Input: part model. Units: mm. Frame: model coordinates. A direction names the side the tool comes from. Round coordinates to 2 decimals unless told otherwise and drop trailing zeros. Order: outer loops, then holes, each group sorted by start corner. A loop starts at its lowest first (then second) coordinate and runs counter-clockwise, first axis right, second up. Notation, with made-up numbers: (30.25, 5.25) -> (50.25, 5.25) arc R19 ccw to (50.25, 27.25) -> close; hole circle Ø5 at (-24, 6). An arc over 180 degrees is marked (long way). Use a Markdown table: item, result.
from build123d import *

# Parameters (mm, degrees)
F0_W     = 2082.8
F0_H     = 914.4
F1_DEPTH = 25.4
F2_W     = 38.1
F2_H     = 88.9
F3_DEPTH = 2082.8
F4_W     = 38.1
F4_H     = 88.9
F5_DEPTH = 838.2
F6_W     = 88.9
F6_H     = 38.1
F7_DEPTH = 1143


# Not quite as in the source:
# - a feature names something its author has since deleted; it is built from what else it names


with BuildPart() as f1:
    # F0 (on Top) → F1 (new body)
    with BuildSketch(Plane.XY):
        with Locations((1041.4, -457.2)):
            Rectangle(F0_W, F0_H)
    extrude(amount=F1_DEPTH)

    # F2 (on face) → F3 (join, through all)
    with BuildSketch(Plane.YZ.offset(2082.8)):
        with Locations((-895.35, -44.45)):
            Rectangle(F2_W, F2_H)
        with Locations((-19.05, -44.45)):
            Rectangle(F2_W, F2_H)
    extrude(amount=-F3_DEPTH)

    # F4 (on face) → F5 (join, through all)
    with BuildSketch(Plane.XZ.offset(38.1)):
        with Locations((19.05, -44.45)):
            Rectangle(F4_W, F4_H)
        with Locations((2063.75, -44.45)):
            Rectangle(F4_W, F4_H)
    extrude(amount=F5_DEPTH)

    # F6 (on face) → F7 (join)
    with BuildSketch(Plane(origin=(0, 0, 0), x_dir=(1, 0, 0), z_dir=(0, 0, -1))):
        with Locations((82.55, 857.25)):
            Rectangle(F6_W, F6_H)
        with Locations((82.55, 57.15)):
            Rectangle(F6_W, F6_H)
        with Locations((2000.25, 57.15)):
            Rectangle(F6_W, F6_H)
        with Locations((2000.25, 857.25)):
            Rectangle(F6_W, F6_H)
    extrude(amount=F7_DEPTH)


solid = f1.part
1) Pull-direction query (Y, two-part tool) for faces 1 (the flat face through (2000, -38.1, -609)), 2 (the flat face through (2082.8, -464, -31)), 3 (the flat face through (82, -76.2, -563)), 4 (the flat face through (2044.7, -452, -45)); classes: +Y half, -Y half, draft (parallel to the pull), parting line (faces both ways), or undercut.
Results found:
| item | result |
|---|---|
| face 1 | +Y half |
| face 2 | draft |
| face 3 | undercut |
| face 4 | undercut |
2) Cut plane A-A on z = -650. Return loops of the section in (x, y), and give its area (3 significant figures).
Results found:
| item | result |
|---|---|
| outline | (38.1, -876.3) -> (127, -876.3) -> (127, -838.2) -> (38.1, -838.2) -> close; (38.1, -76.2) -> (127, -76.2) -> (127, -38.1) -> (38.1, -38.1) -> close; (1955.8, -876.3) -> (2044.7, -876.3) -> (2044.7, -838.2) -> (1955.8, -838.2) -> close; (1955.8, -76.2) -> (2044.7, -76.2) -> (2044.7, -38.1) -> (1955.8, -38.1) -> close |
| area | 13,500 mm² |
3) Cut plane C-C on x = 521.5. Return loops of the section in (y, z), and give its area (3 significant figures).
Results found:
| item | result |
|---|---|
| outline | (-914.4, -88.9) -> (-876.3, -88.9) -> (-876.3, 0) -> (-38.1, 0) -> (-38.1, -88.9) -> (0, -88.9) -> (0, 25.4) -> (-914.4, 25.4) -> close |
| area | 30,000 mm² |
4) Set-up query: faces 5 (the flat face through (82, -38.1, -609)), 6 (the flat face through (82, -876.3, -609)), 7 (the flat face through (1056, -914.4, -33)), 8 (the flat face through (1027, 0, -33)), 9 (the flat face through (38.1, -452, -45)). Return all of +Z, -Z, +X, -X, +Y, -Y with unobstructed straight access to the full face (end or side cutting, diameter ignored); none if empty.
Results found:
| item | result |
|---|---|
| face 5 | -Z, +X, -X, +Y |
| face 6 | -Z, +X, -X, -Y |
| face 7 | +Z, -Z, +X, -X, -Y |
| face 8 | +Z, -Z, +X, -X, +Y |
| face 9 | -Z |
5) Cut plane B-B on y = -240.5. Return loops of the section in (x, z).
Results found:
| item | result |
|---|---|
| outline | (0, -88.9) -> (38.1, -88.9) -> (38.1, 0) -> (2044.7, 0) -> (2044.7, -88.9) -> (2082.8, -88.9) -> (2082.8, 25.4) -> (0, 25.4) -> close |
6) Line query: L1, parallel to X at y = -64, z = -732; L2, parallel to X at y = -382, z = -82; L3, parallel to Z at x = 623, y = -381. Output: solid intervals per line, ascending. Write a range as [from, to].
Results found:
| item | result |
|---|---|
| L1 | x = [38.1, 127], [1955.8, 2044.7] |
| L2 | x = [0, 38.1], [2044.7, 2082.8] |
| L3 | z = [0, 25.4] |
7) Pin query (flat end, axial travel): pin 1 Ø11.5 at (y, z) = (-64.5, -848) entering from -X; pin 2 Ø11.5 at (y, z) = (-50.5, -397.5) entering from +X; pin 3 Ø4 at (x, y) = (1728, -530) entering from -Z. Return the tip coordinate at first contact, or that it passes through.
Results found:
| item | result |
|---|---|
| pin 1 | stops at x = 38.1 |
| pin 2 | stops at x = 2044.7 |
| pin 3 | stops at z = 0 |
